```python
from build123d import *

# Parameters (mm, degrees)
SKETCH_W            = 15
SKETCH_H            = 48
PAD_DEPTH           = 2
SKETCH001_R         = 2.5
POCKET_DEPTH        = 2.001
LINEARPATTERN_COUNT = 2
LINEARPATTERN_PITCH = 24


with BuildPart() as part:
    # Sketch → Pad (new body)
    with BuildSketch(Plane.XZ):
        with Locations((7.5, 24)):
            Rectangle(SKETCH_W, SKETCH_H)
    extrude(amount=PAD_DEPTH)

    # Sketch001 (on Face6 of Pad) → Pocket (cut, through all)
    with BuildSketch(Plane.XZ.offset(2)):
        with Locations((7.5, 7)):
            Circle(SKETCH001_R)
        with Locations((7.5, 17)):
            Circle(SKETCH001_R)
    pocket = extrude(amount=-POCKET_DEPTH, mode=Mode.SUBTRACT)

    # LinearPattern: Pocket ×2
    with Locations(*[(0, 0, i * LINEARPATTERN_PITCH) for i in range(1, LINEARPATTERN_COUNT)]):
        add(pocket, mode=Mode.SUBTRACT)


solid = part.part
```
Geometry check sheet. Reference: the model listing, model coordinates, mm. Round coordinates to 2 decimals unless told otherwise and drop trailing zeros. Loops run counter-clockwise (first coordinate to the right, second up) from the corner with the lowest first, then second, coordinate; pieces in that order, holes last. Notation, with made-up numbers: M -38.75,-34.5 L -32.75,-34.5 A4 cw -32.75,-27.5 Z; hole C -32.5,46.5 d8. An arc over 180 degrees is marked long. Return JSON: item names as keys, results as strings. Group by question number.
(1) Section check B-B, the plane z = 41. Enter the section's corners in (x, y), and give its area (3 significant figures).
(2) Section check A-A, the plane x = 7.5. Enter the section's corners in (y, z), and give its area (3 significant figures).
(3) Scan lines: line 1 along Z through (x, y) = (7.5, -1.3); line 2 along Z through (x, y) = (8.5, -1.05); line 3 along X through (y, z) = (-0.5, 43). Record each from-to range of solid material in increasing order. Write a range as [from, to].
(4) Section check D-D, the plane z = 30. Enter the section's corners in (x, y).
(5) Mould release check, pull along Z, two halves, no side actions. Record for faces 1 (the face through (6.96, -1.01, 38.56)), 2 (the face through (0, -1, 24)), 3 (the face through (7, -1, 48)): pulls with the +Z half, pulls with the -Z half, needs draft (parallel to the pull), parting line crosses it, or undercut.
(6) Section check C-C, the plane y = -0.7. Enter the section's corners in (x, z).
Data:
{
 "1": {"outline": "M 0,-2 L 5,-2 L 5,0 L 0,0 Z; M 10,-2 L 15,-2 L 15,0 L 10,0 Z", "area": "20.0 mm²"},
 "2": {"outline": "M -2,0 L 0,0 L 0,4.5 L -2,4.5 Z; M -2,9.5 L 0,9.5 L 0,14.5 L -2,14.5 Z; M -2,19.5 L 0,19.5 L 0,28.5 L -2,28.5 Z; M -2,33.5 L 0,33.5 L 0,38.5 L -2,38.5 Z; M -2,43.5 L 0,43.5 L 0,48 L -2,48 Z", "area": "56.0 mm²"},
 "3": {"line 1": "[0, 4.5], [9.5, 14.5], [19.5, 28.5], [33.5, 38.5], [43.5, 48]", "line 2": "[0, 4.71], [9.29, 14.71], [19.29, 28.71], [33.29, 38.71], [43.29, 48]", "line 3": "[0, 6], [9, 15]"},
 "4": {"outline": "M 0,-2 L 5.21,-2 L 5.21,0 L 0,0 Z; M 9.79,-2 L 15,-2 L 15,0 L 9.79,0 Z"},
 "5": {"face 1": "undercut", "face 2": "needs draft", "face 3": "pulls with the +Z half"},
 "6": {"outline": "M 0,0 L 15,0 L 15,48 L 0,48 Z; hole C 7.5,7 d5; hole C 7.5,17 d5; hole C 7.5,31 d5; hole C 7.5,41 d5"}
}
